Answer from the drawing. Dimensions are ordinates in mm from the lowest x, y and z of the part. A direction names the side the tool comes from. Coordinates: 2 decimals unless noted, no trailing zeros. Loops run counter-clockwise (first coordinate to the right, second up) from the corner with the lowest first, then second, coordinate; pieces in that order, holes last. Notation, with made-up numbers: M 42,72.5 L 84,72.5 A34 ccw 84,110.5 Z; hole C 22.5,62 d7. An arc over 180 degrees is marked long. Put each result on its own line as item: value.
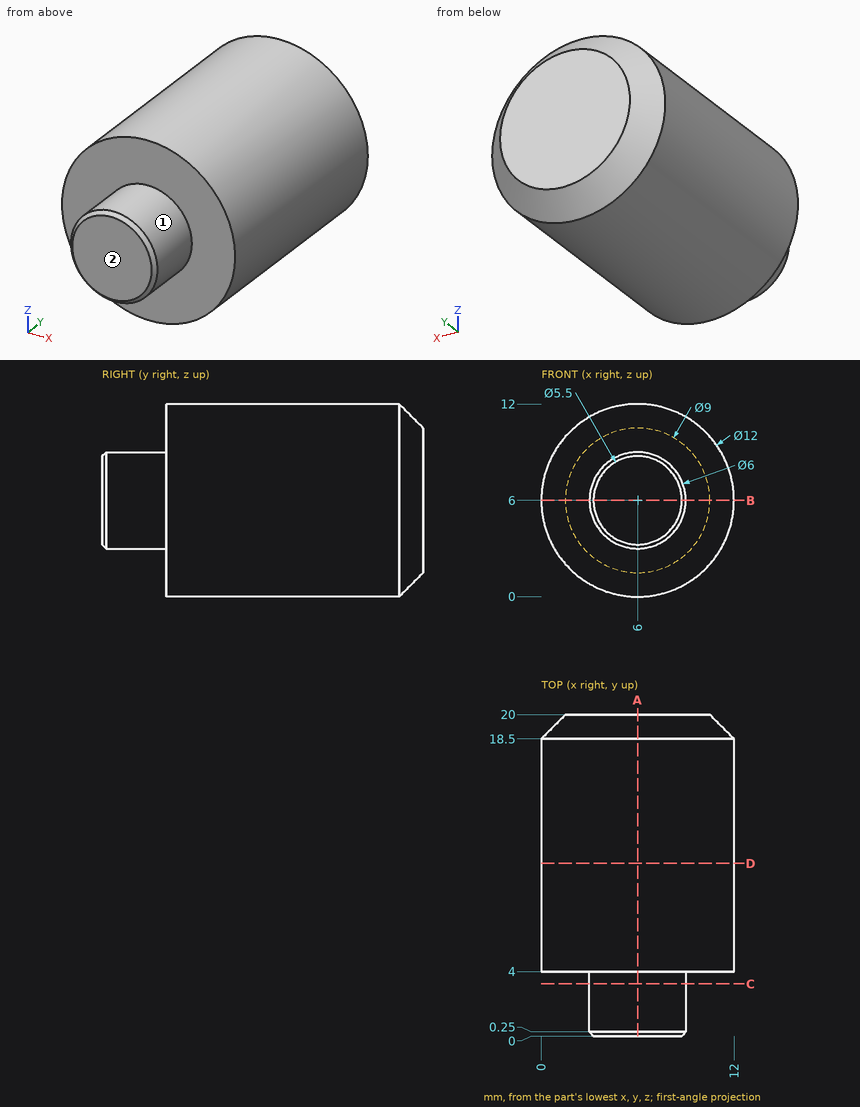
1) Given pin 1 Ø1 at (y, z) = (14.5, 5) entering from +X; pin 2 Ø1.5 at (x, y) = (9.5, 7.5) entering from +Z; pin 3 Ø2 at (y, z) = (11.5, 3) entering from +X, each flat-ended and moving along its own axis, determine where each tip first touches the part or whether it passes through.
Answer list:
pin 1: stops at x = 11.98
pin 2: stops at z = 11.33
pin 3: stops at x = 11.66
2) Find section C-C, the plane y = 3.25. Write down the section's boundary in (x, z), plus the area to 3 significant figures.
Answer list:
outline: C 6,6 d6
area: 28.3 mm^2
3) Which of the six approach directions +Z, -Z, +X, -X, +Y, -Y give full straight-line access (tool end or side, diameter ignored) to the marked faces 1 and 2?
Answer list:
face 1: -Y
face 2: +Z, -Z, +X, -X, -Y
4) Straight lines are drawn through the part: line 1 (Y direction, x = 9.5, z = 4.25); line 2 (Z direction, x = 9.75, y = 8.5); line 3 (X direction, y = 6.5, z = 1.25). For each, find the intervals that lie inside material, in ascending order. Write a range as [from, to].
Answer list:
line 1: y = [4, 20]
line 2: z = [1.32, 10.68]
line 3: x = [2.33, 9.67]
5) Find section B-B, the plane z = 6. Write down the section's boundary in (x, y), plus the area to 3 significant figures.
Answer list:
outline: M 0,4 L 3,4 L 3,0.25 L 3.25,0 L 8.75,0 L 9,0.25 L 9,4 L 12,4 L 12,18.5 L 10.5,20 L 1.5,20 L 0,18.5 Z
area: 214 mm^2
6) Find section A-A, the plane x = 6. Write down the section's boundary in (y, z).
Answer list:
outline: M 0,3.25 L 0.25,3 L 4,3 L 4,0 L 18.5,0 L 20,1.5 L 20,10.5 L 18.5,12 L 4,12 L 4,9 L 0.25,9 L 0,8.75 Z
7) Find section D-D, the plane y = 10.75. Write down the section's boundary in (x, z), plus the area to 3 significant figures.
Answer list:
outline: C 6,6 d12
area: 113 mm^2
